```python
from build123d import *
from OCP.BRepFilletAPI import BRepFilletAPI_MakeChamfer

# Parameters (mm, degrees)
SKETCH1_W           = 36
SKETCH1_H           = 36
SKETCH1_R           = 4
BOSS_EXTRUDE1_DEPTH = 40
CUT_EXTRUDE1_DEPTH  = 36
CHAMFER1_SIZE       = 2
CHAMFER2_SIZE       = 2
CHAMFER2_SIZE2      = 10


with BuildPart() as part:
    # Sketch1 → Boss-Extrude1 (new body)
    with BuildSketch(Plane(origin=(0, 0, 0), x_dir=(1, 0, 0), z_dir=(0, 1, 0))):
        Rectangle(SKETCH1_W, SKETCH1_H)
        with Locations(Location((0, 0, 0), (0, 0, 270))):
            Circle(SKETCH1_R, mode=Mode.SUBTRACT)
    extrude(amount=BOSS_EXTRUDE1_DEPTH)

    # Sketch2 → Cut-Extrude1 (cut)
    with BuildSketch(Plane(origin=(0, 0, 0), x_dir=(1, 0, 0), z_dir=(0, 1, 0))):
        Polygon((-18.585786438, -20), (0, -1.414213562), (18.585786438, -20), (20, -20), (20, -18.585786438), (1.414213562, 0), (20, 18.585786438), (20, 20), (18.585786438, 20), (0, 1.414213562), (-18.585786438, 20), (-20, 20), (-20, 18.585786438), (-1.414213562, 0), (-20, -18.585786438), (-20, -20), align=None)
    extrude(amount=CUT_EXTRUDE1_DEPTH, mode=Mode.SUBTRACT)

    # Chamfer1
    chamfer1_edges = [part.edges().sort_by_distance(p)[0] for p in [
        (-18, 38, -18),
        (18, 38, -18),
        (-18, 38, 18),
        (18, 38, 18),
    ]]
    chamfer(chamfer1_edges, length=CHAMFER1_SIZE)

    # Chamfer2: one chamfer whose edges measure the first distance from different faces: ONE call of the kernel's chamfer builder (chamfer() names one face for all edges)
    chamfer2_edges_1 = [part.edges().sort_by_distance(p)[0] for p in [
        (0, 0, -18),
    ]]
    chamfer2_side_1 = [part.faces().sort_by_distance(p)[0] for p in [
        (0, 0, -12.666463052),
    ]]
    chamfer2_edges_2 = [part.edges().sort_by_distance(p)[0] for p in [
        (18, 0, 0),
    ]]
    chamfer2_side_2 = [part.faces().sort_by_distance(p)[0] for p in [
        (12.666463052, 0, 0),
    ]]
    chamfer2_edges_3 = [part.edges().sort_by_distance(p)[0] for p in [
        (0, 0, 18),
    ]]
    chamfer2_side_3 = [part.faces().sort_by_distance(p)[0] for p in [
        (0, 0, 12.666463052),
    ]]
    chamfer2_edges_4 = [part.edges().sort_by_distance(p)[0] for p in [
        (-18, 0, 0),
    ]]
    chamfer2_side_4 = [part.faces().sort_by_distance(p)[0] for p in [
        (-12.666463052, 0, 0),
    ]]
    chamfer2 = BRepFilletAPI_MakeChamfer(part.part.solid().wrapped)
    for e in chamfer2_edges_1:
        chamfer2.Add(CHAMFER2_SIZE, CHAMFER2_SIZE2, e.wrapped, chamfer2_side_1[0].wrapped)  # the first distance lies on this face
    for e in chamfer2_edges_2:
        chamfer2.Add(CHAMFER2_SIZE, CHAMFER2_SIZE2, e.wrapped, chamfer2_side_2[0].wrapped)  # the first distance lies on this face
    for e in chamfer2_edges_3:
        chamfer2.Add(CHAMFER2_SIZE, CHAMFER2_SIZE2, e.wrapped, chamfer2_side_3[0].wrapped)  # the first distance lies on this face
    for e in chamfer2_edges_4:
        chamfer2.Add(CHAMFER2_SIZE, CHAMFER2_SIZE2, e.wrapped, chamfer2_side_4[0].wrapped)  # the first distance lies on this face
    add(Compound.cast(chamfer2.Shape()), mode=Mode.REPLACE)


solid = part.part
```
Geometry check sheet. Reference: the model listing, model coordinates, mm. A direction names the side the tool comes from. Coordinates: 2 decimals unless noted, no trailing zeros. Order: outer loops, then holes, each group sorted by start corner. A loop starts at its lowest first (then second) coordinate and runs counter-clockwise, first axis right, second up.
Q1. Sectioned sample at D-D on x = 8. Record the cut outline in (y, z), and give its area (3 significant figures).
Reply:
outline: (0, -16) - (10, -18) - (40, -18) - (40, 18) - (10, 18) - (0, 16) - (0, 9.41) - (36, 9.41) - (36, 6.59) - (0, 6.59) - (0, -6.59) - (36, -6.59) - (36, -9.41) - (0, -9.41) - close
area: 1,220 mm2
Q2. Sectioned sample at C-C on y = 27. Record the cut outline in (x, z), and give its area (3 significant figures).
Reply:
outline: (-18, -16) - (-17.71, -16.29) - (-3.45, -2.03) arc R4 cw to (-3.45, 2.03) - (-17.71, 16.29) - (-18, 16) - close; (-16.29, -17.71) - (-16, -18) - (16, -18) - (16.29, -17.71) - (2.03, -3.45) arc R4 cw to (-2.03, -3.45) - close; (-16.29, 17.71) - (-2.03, 3.45) arc R4 cw to (2.03, 3.45) - (16.29, 17.71) - (16, 18) - (-16, 18) - close; (3.45, -2.03) - (17.71, -16.29) - (18, -16) - (18, 16) - (17.71, 16.29) - (3.45, 2.03) arc R4 cw to start
area: 1,080 mm2
Q3. Sectioned sample at A-A on x = 0. Record the cut outline in (y, z), and give its area (3 significant figures).
Reply:
outline: (0, -16) - (10, -18) - (40, -18) - (40, -4) - (0, -4) - close; (0, 4) - (40, 4) - (40, 18) - (10, 18) - (0, 16) - close
area: 1,100 mm2
Q4. Tool access check on faces 1 (the face through (-17, 5, 0)), 2 (the face through (10, 36, 10)). Record the directions out of +Z, -Z, +X, -X, +Y, -Y that give a thin tool (end or side, any length) a straight path to the whole face; none if there is none.
Reply:
face 1: +Z, -Z, -X, -Y
face 2: -Y
Q5. Draft check along X on faces 3 (the face through (0, 5, 17)), 4 (the face through (-16.11, 27.69, -17.89)), 5 (the face through (9.062, 17.748, 10.477)). Enter one of: released by +X, released by -X, zero draft, split by the parting line, or undercut.
Reply:
face 3: zero draft
face 4: released by -X
face 5: undercut
Q6. Sectioned sample at B-B on z = 0. Record the cut outline in (x, y).
Reply:
outline: (-18, 10) - (-16, 0) - (-4, 0) - (-4, 40) - (-18, 40) - close; (4, 0) - (16, 0) - (18, 10) - (18, 40) - (4, 40) - close
Q7. Thickness scan on probe 1 along Z at (x, y) = (0, 30); probe 2 along X at (y, z) = (34.5, -11). Record the ranges inside material, lowest first.
Reply:
probe 1: z = -18 to -4, 4 to 18
probe 2: x = -18 to -12.41, -9.59 to 9.59, 12.41 to 18
